Read the model definition and answer for the solid it produces. Units are mm, in the model's axes. A direction names the side the tool comes from. Coordinates: 2 decimals unless noted, no trailing zeros. Loops run counter-clockwise (first coordinate to the right, second up) from the corner with the lowest first, then second, coordinate; pieces in that order, holes last.
from build123d import *

# Parameters (mm, degrees)
SKETCH_2_W             = 38
SKETCH_2_H             = 39
EXTRUDE_1_DEPTH        = 2
CHAMFER_3_SIZE         = 1
SKETCH_7_R             = 4.25
CUT_EXTRUDE_3_DEPTH    = 10
SKETCH_8_W             = 2
SKETCH_8_H             = 39
CUT_EXTRUDE_4_DEPTH    = 10
FILLET_3_R             = 2
SKETCH_9_R             = 2
EXTRUDE_1_2_DEPTH      = 26
SKETCH_10_W            = 3
SKETCH_10_H            = 39
CUT_EXTRUDE_1_DEPTH    = 10
FILLET_5_R             = 2
CHAMFER_5_SIZE         = 0.5
HOLE_WIZARD_M2_5_3_D   = 2.05
HOLE_WIZARD_M2_1_D     = 1.6
HOLE_WIZARD_M2_1_DEPTH = 7
HOLE_WIZARD_M2_1_TIP   = 0.480688495
CUT_EXTRUDE_2_DEPTH    = 10
SKETCH_24_W            = 71.290640242
SKETCH_24_H            = 51.144653494
CUT_EXTRUDE_3_2_DEPTH  = 10
SKETCH_25_R            = 6.539265834
CUT_EXTRUDE_4_2_DEPTH  = 32
HOLE_WIZARD_M2_2_D     = 1.6
HOLE_WIZARD_M2_2_DEPTH = 7
HOLE_WIZARD_M2_2_TIP   = 0.480688495
FILLET_6_SIZE          = 0.5


with BuildPart() as part:
    # 草图2 → Extrude 1 (new body)
    with BuildSketch(Plane.XY):
        Rectangle(SKETCH_2_W, SKETCH_2_H)
    extrude(amount=EXTRUDE_1_DEPTH)

    # 倒角3
    chamfer_3_edges = [part.edges().sort_by_distance(p)[0] for p in [
        (-19, 19.5, 1),
        (-19, -19.5, 1),
    ]]
    chamfer(chamfer_3_edges, length=CHAMFER_3_SIZE)

    # 草图7 → Cut-Extrude 3 (cut)
    with BuildSketch(Plane.XY.offset(2)):
        with Locations((2, 0)):
            Circle(SKETCH_7_R)
    extrude(amount=-CUT_EXTRUDE_3_DEPTH, mode=Mode.SUBTRACT)

    # 草图8 → Cut-Extrude 4 (cut)
    with BuildSketch(Plane.XY.offset(2)):
        with Locations((-18, 0)):
            Rectangle(SKETCH_8_W, SKETCH_8_H)
    extrude(amount=-CUT_EXTRUDE_4_DEPTH, mode=Mode.SUBTRACT)

    # 圆角3
    fillet_3_edges = [part.edges().sort_by_distance(p)[0] for p in [
        (-17, 19.5, 1),
        (-17, -19.5, 1),
    ]]
    fillet(fillet_3_edges, radius=FILLET_3_R)

    # 草图9 → Extrude 1 2 (add)
    with BuildSketch(Plane.XY.offset(2)):
        with Locations((-15, 17.5)):
            Circle(SKETCH_9_R)
        with Locations((-15, -17.5)):
            Circle(SKETCH_9_R)
    extrude_1_2 = extrude(amount=EXTRUDE_1_2_DEPTH)

    # 镜向1: Extrude 1 2 across plane
    add(extrude_1_2.mirror(Plane.ZX))

    # 草图10 → 切除-拉伸1 (cut)
    with BuildSketch(Plane(origin=(0, 0, 0), x_dir=(-1, 0, 0), z_dir=(0, 0, -1))):
        with Locations((-17.5, 0)):
            Rectangle(SKETCH_10_W, SKETCH_10_H)
    extrude(amount=-CUT_EXTRUDE_1_DEPTH, mode=Mode.SUBTRACT)

    # 圆角5
    fillet_5_edges = [part.edges().sort_by_distance(p)[0] for p in [
        (16, -19.5, 1),
        (16, 19.5, 1),
    ]]
    fillet(fillet_5_edges, radius=FILLET_5_R)

    # 倒角5
    chamfer_5_edges = [part.edges().sort_by_distance(p)[0] for p in [
        (-17, -17.5, 28),
        (-17, 17.5, 28),
        (15.414213562, 18.914213562, 0),
        (16, 0, 0),
        (-0.5, 19.5, 0),
        (15.414213562, -18.914213562, 0),
        (-16.414213562, 18.914213562, 0),
        (-0.5, -19.5, 0),
        (-17, 0, 0),
        (-16.414213562, -18.914213562, 0),
    ]]
    chamfer(chamfer_5_edges, length=CHAMFER_5_SIZE)

    # M2.5 螺纹孔3 (through all)
    with Locations(Plane(origin=(9.5, 15.5, 0), x_dir=(-1, 0, 0), z_dir=(0, 0, -1))):
        with Locations((0, 0), (15, 0), (0, -31), (15, -31)):
            Hole(HOLE_WIZARD_M2_5_3_D / 2)

    # M2 螺纹孔1
    with Locations(Plane(origin=(-15, 17.5, 28), x_dir=(1, 0, 0), z_dir=(0, 0, 1))):
        with Locations((0, 0), (0, -35)):
            Hole(HOLE_WIZARD_M2_1_D / 2, depth=HOLE_WIZARD_M2_1_DEPTH)
            with Locations((0, 0, -(HOLE_WIZARD_M2_1_DEPTH + HOLE_WIZARD_M2_1_TIP / 2))):  # 118° drill point
                Cone(0, HOLE_WIZARD_M2_1_D / 2, HOLE_WIZARD_M2_1_TIP, mode=Mode.SUBTRACT)

    # 草图23 → 切除-拉伸2 (cut)
    with BuildSketch(Plane(origin=(0, 0, 0), x_dir=(-1, 0, 0), z_dir=(0, 0, -1))):
        with BuildLine():
            Line((-0.95, 16.2), (-0.95, 9.8))
            ThreePointArc((-0.95, 9.8), (-2, 8.75), (-3.05, 9.8))
            Line((-3.05, 9.8), (-3.05, 16.2))
            ThreePointArc((-3.05, 16.2), (-2, 17.25), (-0.95, 16.2))
        make_face()
    cut_extrude_2 = extrude(amount=-CUT_EXTRUDE_2_DEPTH, mode=Mode.SUBTRACT)

    # 镜向2: 切除-拉伸2 across plane
    add(cut_extrude_2.mirror(Plane.ZX), mode=Mode.SUBTRACT)

    # 草图24 → Cut-Extrude 3 2 (cut)
    with BuildSketch(Plane.XY.offset(2)):
        Rectangle(SKETCH_24_W, SKETCH_24_H)
    extrude(amount=-CUT_EXTRUDE_3_2_DEPTH, mode=Mode.SUBTRACT)


with BuildPart() as cut_extrude_3_2_piece_1:
    # of the separate pieces the step leaves, piece 1, a body of its own (cut_extrude_3_2_pieces)
    add(part.part.solids().sort_by_distance((-13, 17.5, 27.5))[0])

    # 草图25 → Cut-Extrude 4 2 (cut)
    with BuildSketch(Plane(origin=(0, 0, 2), x_dir=(-1, 0, 0), z_dir=(0, 0, -1))):
        with Locations((15, 17.5)):
            Circle(SKETCH_25_R)
    extrude(amount=-CUT_EXTRUDE_4_2_DEPTH, mode=Mode.SUBTRACT)


with BuildPart() as cut_extrude_3_2_piece_2:
    # of the separate pieces the step leaves, piece 2, a body of its own (cut_extrude_3_2_pieces)
    add(part.part.solids().sort_by_distance((-13, -17.5, 2))[0])

    # M2 螺纹孔2
    with Locations(Plane(origin=(-15, -17.5, 2), x_dir=(-1, 0, 0), z_dir=(0, 0, -1))):
        with Locations((0, 0)):
            Hole(HOLE_WIZARD_M2_2_D / 2, depth=HOLE_WIZARD_M2_2_DEPTH)
            with Locations((0, 0, -(HOLE_WIZARD_M2_2_DEPTH + HOLE_WIZARD_M2_2_TIP / 2))):  # 118° drill point
                Cone(0, HOLE_WIZARD_M2_2_D / 2, HOLE_WIZARD_M2_2_TIP, mode=Mode.SUBTRACT)

    # 圆角6
    # a fillet whose section is not a circle: 0.5 mm, written as the material it takes off along each edge
    with BuildSketch(Plane(origin=(-15, -17.5, 2), x_dir=(1, 0, 0), z_dir=(0, -1, 0))) as fillet_6_piece_1:
        with BuildLine():
            Bezier((2, FILLET_6_SIZE), (2, 0), (2 - FILLET_6_SIZE, 0), weights=[1, 0.035355339, 1])
            Line((2 - FILLET_6_SIZE, 0), (2, 0))
            Line((2, 0), (2, FILLET_6_SIZE))
        make_face()
    revolve(axis=Axis((-15, -17.5, 2), (0, 0, 1)), mode=Mode.SUBTRACT)


solid = cut_extrude_3_2_piece_2.part
Item 1: A cutting plane is placed at A-A on z = 21.5. Determine the outline of the cut face in (x, y).
Numbers:
outline: circle Ø4 at (-15, -17.5); hole circle Ø1.6 at (-15, -17.5)
Item 2: Find the intervals of material crossed by line 1 along Y through (x, z) = (-15, 25.25); line 2 along Y through (x, z) = (-14.3, 25); line 3 along X through (y, z) = (-17.25, 6.5), in increasing order.
Numbers:
line 1: y = -19.5 to -18.3, -16.7 to -15.5
line 2: y = -19.37 to -17.89, -17.11 to -15.63
line 3: x = -16.98 to -15.76, -14.24 to -13.02
Item 3: A cutting plane is placed at B-B on z = 10.5. Determine the outline of the cut face in (x, y).
Numbers:
outline: circle Ø4 at (-15, -17.5)
Item 4: Determine the mould class of faces 4 (the face through (-14, -18, 2)), 5 (the face through (-14.872, -17.553, 20.603)), 6 (the face through (-15.26, -15.517, 14.825)) for opening direction X: released by +X, released by -X, zero draft, split by the parting line, or undercut.
Numbers:
face 4: zero draft
face 5: undercut
face 6: split by the parting line
Item 5: Which of the six approach directions +Z, -Z, +X, -X, +Y, -Y give full straight-line access (tool end or side, diameter ignored) to faces 1 (the face through (-14, -18, 28)), 2 (the face through (-15.63, -17.99, 5.55)), 3 (the face through (-14.37, -17.99, 24.45))?
Numbers:
face 1: +Z, +X, -X, +Y, -Y
face 2: -Z
face 3: +Z
Item 6: Given pin 1 (2 mm diameter, centred on x = -15, y = -17.5, fed in from +Z), flat-ended and moving along its own axis, determine where the tip first touches the part or whether it passes through.
Numbers:
pin 1: stops at z = 28
